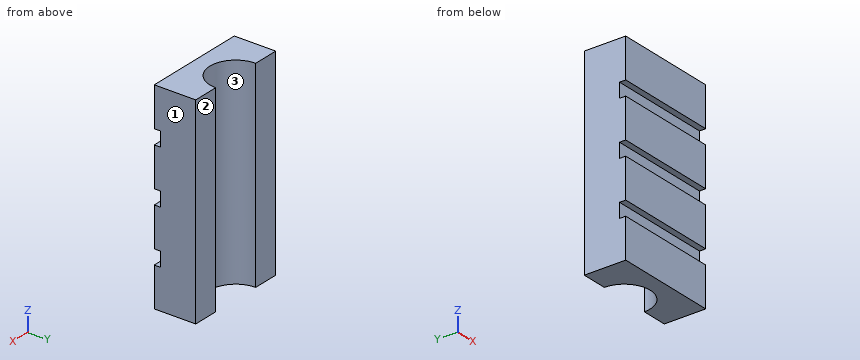
```python
from build123d import *

# Parameters (mm, degrees)
SKETCH1_W           = 50
SKETCH1_H           = 97
BOSS_EXTRUDE1_DEPTH = 20
SKETCH2_R           = 12.5
CUT_EXTRUDE1_DEPTH  = 100
SKETCH3_W           = 50
SKETCH3_H           = 7
CUT_EXTRUDE2_DEPTH  = 3


with BuildPart() as part:
    # Sketch1 → Boss-Extrude1 (new body)
    with BuildSketch(Plane(origin=(0, 0, 0), x_dir=(1, 0, 0), z_dir=(0, 1, 0))):
        with Locations((25, -48.5)):
            Rectangle(SKETCH1_W, SKETCH1_H)
    extrude(amount=BOSS_EXTRUDE1_DEPTH)

    # Sketch2 → Cut-Extrude1 (cut)
    with BuildSketch(Plane.XY.offset(97)):
        with Locations((25, 20)):
            Circle(SKETCH2_R)
    extrude(amount=-CUT_EXTRUDE1_DEPTH, mode=Mode.SUBTRACT)

    # Sketch3 → Cut-Extrude2 (cut)
    with BuildSketch(Plane.XZ):
        with Locations((25, 74.5)):
            Rectangle(SKETCH3_W, SKETCH3_H)
        with Locations((25, 48.5)):
            Rectangle(SKETCH3_W, SKETCH3_H)
        with Locations((25, 22.5)):
            Rectangle(SKETCH3_W, SKETCH3_H)
    extrude(amount=-CUT_EXTRUDE2_DEPTH, mode=Mode.SUBTRACT)


solid = part.part
```
Build history of the part. All positions in model axes, mm. Face numbers are marked on the shaded views. Give positions to 0.01 mm unless a question says otherwise; leave off trailing zeros. Order: outer loops, then holes, each group sorted by start corner. A loop starts at its lowest first (then second) coordinate and runs counter-clockwise, first axis right, second up. Notation, with made-up numbers: M 7,84.25 L 12,84.25 A17 cw 12,109.25 Z; hole C 71,89.5 d9. An arc over 180 degrees is marked long. Write item = value, one per line. Start each with the question number.
(1) Slice it at B-B on x = 25.5. Write the cut outline in (y, z).
(2) Probe L1, parallel to Z at x = 17, y = 2.5; L2, parallel to X at y = 10.5, z = 20.5; L3, parallel to X at y = 12.5, z = 64.5. List the from-to ranges inside material, lowest first. Write a range as [from, to].
(3) Slice it at D-D on x = 44.5. Write the cut outline in (y, z).
(4) Pin check, flat tips, straight feed: pin 1 Ø2 at (x, z) = (36.5, 23) entering from -Y; pin 2 Ø5 at (x, z) = (17, 42.5) entering from +Y; pin 3 Ø1 at (x, z) = (21.5, 31.5) entering from +Y. Stop position of each tip, or through.
(5) Slice it at A-A on y = 12.5. Write the cut outline in (x, z), plus the area to 3 significant figures.
(6) Two-plate mould, pull along X, no slides. Class the marked faces 1, 2 and 3: released by +X, released by -X, zero draft, split by the parting line, or undercut.
(7) Slice it at C-C on z = 91.5. Write the cut outline in (x, y).
Responses:
q1.outline = M 0,0 L 7.51,0 L 7.51,97 L 0,97 L 0,78 L 3,78 L 3,71 L 0,71 L 0,52 L 3,52 L 3,45 L 0,45 L 0,26 L 3,26 L 3,19 L 0,19 Z
q2.L1 = [0, 19], [26, 45], [52, 71], [78, 97]
q2.L2 = [0, 16.88], [33.12, 50]
q2.L3 = [0, 15], [35, 50]
q3.outline = M 0,0 L 20,0 L 20,97 L 0,97 L 0,78 L 3,78 L 3,71 L 0,71 L 0,52 L 3,52 L 3,45 L 0,45 L 0,26 L 3,26 L 3,19 L 0,19 Z
q4.pin_1 = 3
q4.pin_2 = 13.22
q4.pin_3 = 8.16
q5.outline = M 0,0 L 15,0 L 15,97 L 0,97 Z; M 35,0 L 50,0 L 50,97 L 35,97 Z
q5.area = 2,910 mm2
q6.face_1 = released by +X
q6.face_2 = zero draft
q6.face_3 = undercut
q7.outline = M 0,0 L 50,0 L 50,20 L 37.5,20 A12.5 cw 12.5,20 L 0,20 Z
